```python
from build123d import *

# Parameters (mm, degrees)
CROQUIS1_W              = 50.8
CROQUIS1_H              = 6.31
SALIENTE_EXTRUIR1_DEPTH = 228.75
CROQUIS2_W              = 50.8
CROQUIS2_H              = 6.31
SALIENTE_EXTRUIR2_DEPTH = 801.67
CROQUIS3_W              = 50.8
CROQUIS3_H              = 6.31
SALIENTE_EXTRUIR3_DEPTH = 552.5
CROQUIS4_W              = 50.8
CROQUIS4_H              = 6.31
SALIENTE_EXTRUIR4_DEPTH = 314.39
CROQUIS6_W              = 50.8
CROQUIS6_H              = 6.31
SALIENTE_EXTRUIR5_DEPTH = 10
CROQUIS7_W              = 50.8
CROQUIS7_H              = 6.31
SALIENTE_EXTRUIR6_DEPTH = 50.8
CROQUIS12_R             = 6.5
CORTAR_EXTRUIR3_DEPTH   = 10
CROQUIS13_R             = 5
CORTAR_EXTRUIR4_DEPTH   = 35


with BuildPart() as part:
    # Croquis1 → Saliente-Extruir1 (new body)
    with BuildSketch(Plane.XY):
        Rectangle(CROQUIS1_W, CROQUIS1_H)
    extrude(amount=SALIENTE_EXTRUIR1_DEPTH)

    # Croquis2 → Saliente-Extruir2 (add)
    with BuildSketch(Plane.XZ.offset(3.155)):
        with Locations((0, 225.595)):
            Rectangle(CROQUIS2_W, CROQUIS2_H)
    extrude(amount=SALIENTE_EXTRUIR2_DEPTH)

    # Croquis3 → Saliente-Extruir3 (add)
    with BuildSketch(Plane.XY.offset(228.75)):
        with Locations((0, -801.67)):
            Rectangle(CROQUIS3_W, CROQUIS3_H)
    extrude(amount=SALIENTE_EXTRUIR3_DEPTH)

    # Croquis4 → Saliente-Extruir4 (add)
    with BuildSketch(Plane(origin=(0, -798.515, 0), x_dir=(1, 0, 0), z_dir=(0, 1, 0))):
        with Locations((0, -778.095)):
            Rectangle(CROQUIS4_W, CROQUIS4_H)
    extrude(amount=SALIENTE_EXTRUIR4_DEPTH)

    # Croquis6 → Saliente-Extruir5 (add)
    with BuildSketch(Plane(origin=(0, -484.125, 0), x_dir=(1, 0, 0), z_dir=(0, 1, 0))):
        with Locations((0, -778.095)):
            Rectangle(CROQUIS6_W, CROQUIS6_H)
    extrude(amount=SALIENTE_EXTRUIR5_DEPTH)

    # Croquis7 → Saliente-Extruir6 (add)
    with BuildSketch(Plane(origin=(0, 3.155, 0), x_dir=(1, 0, 0), z_dir=(0, 1, 0))):
        with Locations((0, -3.155)):
            Rectangle(CROQUIS7_W, CROQUIS7_H)
    extrude(amount=-SALIENTE_EXTRUIR6_DEPTH)

    # Croquis12 → Cortar-Extruir3 (cut)
    with BuildSketch(Plane.XY.offset(781.25)):
        with Locations((0, -521.625)):
            Circle(CROQUIS12_R)
        with Locations((0, -490.625)):
            Circle(CROQUIS12_R)
    extrude(amount=-CORTAR_EXTRUIR3_DEPTH, mode=Mode.SUBTRACT)

    # Croquis13 → Cortar-Extruir4 (cut)
    with BuildSketch(Plane.XY.offset(781.25)):
        with Locations((0, -718.315)):
            Circle(CROQUIS13_R)
    extrude(amount=-CORTAR_EXTRUIR4_DEPTH, mode=Mode.SUBTRACT)


solid = part.part
```
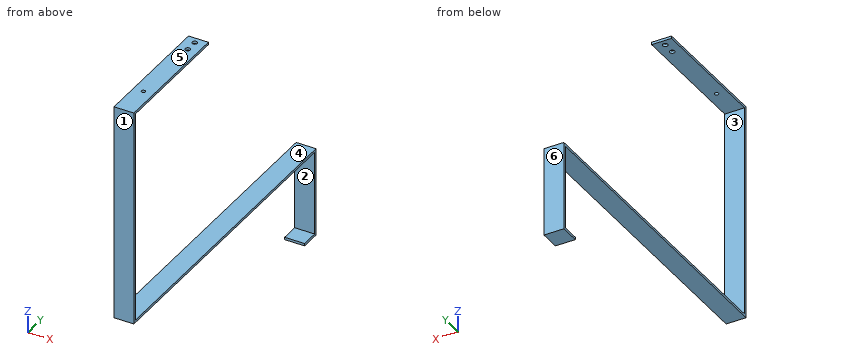
CAD build for the part. Positions are in the model's coordinates, mm. Face numbers are marked on the shaded views. A direction names the side the tool comes from. Coordinates: 2 decimals unless noted, no trailing zeros. Write each loop counter-clockwise with the first axis right and the second up, starting at its lowest first coordinate (ties: lowest second). Pieces come first, ordered by that corner, then holes. Notation, with made-up numbers: (-18.5, 88) -> (8.5, 88) arc R5 cw to (8.5, 97) -> close; hole circle Ø10 at (24, -1.75). An arc over 180 degrees is marked (long way). Use CSV: the item, a comma, the result in double quotes. Start each with the question number.
Item 1: Band-saw the part on A-A, the plane y = -581.5. Write the cut outline in (x, z), plus the area to 3 significant figures.
Item 2: Wall check: probe 1 along Y at (x, z) = (0, 778) (3 decimals); probe 2 along Z at (x, y) = (-9, -598.5); probe 3 along Z at (x, y) = (-22, -453.5). Give the ranges that are in metal, low to high.
Item 3: Tool access for the marked faces 1, 2 and 3: list every direction of +Z, -Z, +X, -X, +Y, -Y with a clear straight run to the whole face (end or side of a thin tool).
Item 4: Drop flat-ended pins along their axis: P1, Ø10.5, axis at x = 0, y = -490.625, coming from the +Z side; P2, Ø5, axis at x = 14.5, z = 531, coming from the +Y side (3 decimals); P3, Ø8, axis at x = 0, y = -521.625, coming from the -Z side. Give the stop position or say it passes through.
Item 5: Two-plate mould, pull along Z, no slides. Class the marked faces 4, 5 and 6: +Z half, -Z half, draft (parallel to the pull), parting line (faces both ways), or undercut.
Item 6: Band-saw the part on C-C, the plane y = -232.5. Write the cut outline in (x, z).
Item 7: Band-saw the part on B-B, the plane z = 728.5. Write the cut outline in (x, y) (3 decimals).
Response values:
1,outline,"(-25.4, 222.44) -> (25.4, 222.44) -> (25.4, 228.75) -> (-25.4, 228.75) -> close; (-25.4, 774.94) -> (25.4, 774.94) -> (25.4, 781.25) -> (-25.4, 781.25) -> close"
1,area,"641 mm2"
2,probe 1,"y = -804.825 to -723.315, -713.315 to -528.125, -515.125 to -497.125, -484.125 to -474.125"
2,probe 2,"z = 222.44 to 228.75, 774.94 to 781.25"
2,probe 3,"z = 222.44 to 228.75"
3,face 1,"+Z, -Z, +X, -X, -Y"
3,face 2,"+X, -X, -Y"
3,face 3,"+X, -X, +Y"
4,P1,"stops at z = 228.75"
4,P2,"stops at y = -798.515"
4,P3,"stops at z = 222.44"
5,face 4,"undercut"
5,face 5,"+Z half"
5,face 6,"draft"
6,outline,"(-25.4, 222.44) -> (25.4, 222.44) -> (25.4, 228.75) -> (-25.4, 228.75) -> close"
7,outline,"(-25.4, -804.825) -> (25.4, -804.825) -> (25.4, -798.515) -> (-25.4, -798.515) -> close"
